Autodesk Inventor part; units mm, degrees
ref_plane "YZ Plane" through (0, 0, 0) normal (1, 0, 0) x (0, 1, 0)
ref_plane "XZ Plane" through (0, 0, 0) normal (0, 1, 0) x (-1, 0, 0)
ref_plane "XY Plane" through (0, 0, 0) normal (0, 0, 1) x (1, 0, 0)
sketch "Sketch3" plane through (0, 0, 0) normal (0, 0, 1) x (1, 0, 0)
  circle A0 centre (0, 0) radius 4.45
  dimension "d11" = 8.9
extrude "Extrusion3" add sketch "Sketch3" along normal blind 6
sketch "Sketch4" plane through (0, 0, 6) normal (0, 0, 1) x (1, 0, 0)
  circle A0 centre (0, 0) radius 30
  dimension "d14" = 60
extrude "Extrusion4" add sketch "Sketch4" along normal blind 8
ref_plane "Work Plane2" through (0, 0, 8) normal (0, 0, 1) x (1, 0, 0)
ref_plane "Work Plane1" through (0, 0, 10) normal (0, 0, 1) x (1, 0, 0)
sketch "Sketch5" plane through (0, 0, 8) normal (0, 0, 1) x (1, 0, 0)
  circle A0 centre (0, 0) radius 28.5
  circle A1 centre (0, 0) radius 30
  dimension "d17" = 57
  dimension "d18" = 60
extrude "Extrusion5" cut sketch "Sketch5" along normal mid plane 2
mirror "Mirror1" about plane through (0, 0, 10) normal (0, 0, 1) of "Extrusion5"
sketch "Sketch7" plane through (0, 0, 0) normal (0, 0, -1) x (-1, 0, 0)
  line L0 (-3.4063, 0) -> (1.7033, -2.95)
  line L1 (1.7033, -2.95) -> (1.7033, 2.95)
  line L2 (-3.4063, 0) -> (1.7033, 2.95)
  dimension "d29" = 5.9
  dimension "d30" = 5.9
  dimension "d34" = 5.9
extrude "Extrusion7" add sketch "Sketch7" along normal blind 22
sketch "Sketch8" plane through (-1.7033, -2.95, 0) normal (-1, 0, 0) x (0, 0, 1)
  line L0 (0, 2.95) -> (-22, 2.95)
  circle A0 centre (-20.8375, 2.95) radius 0.75
  dimension "d37" = 1.5
extrude "Extrusion8" cut sketch "Sketch8" against normal blind 12
ref_plane "Work Plane3" through (0, 0, 10) normal (0, 0, 1) x (1, 0, 0)
ref_plane "Work Plane4" through (0, 0, 12) normal (0, 0, 1) x (1, 0, 0)
equation "\"d29\" = d34"
equation "\"d30\" = d34"
properties part number "PulleyAdapterLong" material "ABS Plastic"
Verification items for the finished model (mm, model axes). A direction names the side the tool comes from. Coordinates: 2 decimals unless noted, no trailing zeros. Order: outer loops, then holes, each group sorted by start corner. A loop starts at its lowest first (then second) coordinate and runs counter-clockwise, first axis right, second up.
1. Release check for a two-part mould opening along Z. For faces 1 (the face through (0, 0, 14)), 2 (the face through (11, -27, 9)), 3 (the face through (-29.97, -1.32, 13.49)) record: +Z half, -Z half, draft (parallel to the pull), parting line (faces both ways), or undercut.
Results found:
face 1: +Z half
face 2: undercut
face 3: draft
2. Set-up check for faces 4 (the face through (-1.703, 0, -11)), 5 (the face through (0.887, 1.454, -10.846)), 6 (the face through (0.887, -1.454, -10.846)), 7 (the face through (-11, -27, 13)): record each of +Z, -Z, +X, -X, +Y, -Y from which the full face is reachable in a straight line by a thin tool's end or side.
Results found:
face 4: -Z, -X, +Y, -Y
face 5: -Z, +X, +Y
face 6: -Z, +X, -Y
face 7: none
3. Go/stop test with flat-tipped pins: pin 1 Ø10 at (y, z) = (-2.5, -2.5) entering from +X; pin 2 Ø8 at (y, z) = (-16, 6.5) entering from -X; pin 3 Ø2 at (y, z) = (0, -20.84) entering from -X; pin 4 Ø2.5 at (x, y) = (1.5, -2) entering from -Z. Record where each tip stops, or that it passes through.
Results found:
pin 1: stops at x = 4.45
pin 2: stops at x = -27.5
pin 3: stops at x = -1.7
pin 4: stops at z = -22
4. Sectioned sample at C-C, the plane y = -20. Record the cut outline in (x, z).
Results found:
outline: (-22.36, 6) - (22.36, 6) - (22.36, 7) - (20.3, 7) - (20.3, 9) - (22.36, 9) - (22.36, 11) - (20.3, 11) - (20.3, 13) - (22.36, 13) - (22.36, 14) - (-22.36, 14) - (-22.36, 13) - (-20.3, 13) - (-20.3, 11) - (-22.36, 11) - (-22.36, 9) - (-20.3, 9) - (-20.3, 7) - (-22.36, 7) - close
5. Scan lines: line 1 (Z direction, x = 1, y = 0); line 2 (Z direction, x = -5, y = 20.5); line 3 (Y direction, x = 6, z = 11.5). Record each from-to range of solid material in increasing order.
Results found:
line 1: z = -22 to -21.59, -20.09 to 14
line 2: z = 6 to 14
line 3: y = -27.86 to 27.86
6. Sectioned sample at B-B, the plane z = -10.5. Record the cut outline in (x, y), and give its area (3 significant figures).
Results found:
outline: (-1.7, -2.95) - (3.41, 0) - (-1.7, 2.95) - close
area: 15.1 mm2
7. Sectioned sample at A-A, the plane x = -10.5. Record the cut outline in (y, z).
Results found:
outline: (-28.1, 6) - (28.1, 6) - (28.1, 7) - (26.5, 7) - (26.5, 9) - (28.1, 9) - (28.1, 11) - (26.5, 11) - (26.5, 13) - (28.1, 13) - (28.1, 14) - (-28.1, 14) - (-28.1, 13) - (-26.5, 13) - (-26.5, 11) - (-28.1, 11) - (-28.1, 9) - (-26.5, 9) - (-26.5, 7) - (-28.1, 7) - close
